from build123d import *

# Parameters (mm, degrees)
SKETCH1_R           = 50
BOSS_EXTRUDE1_DEPTH = 7
SKETCH2_R           = 2.5
BOSS_EXTRUDE2_DEPTH = 12.6
CIRPATTERN1_COUNT   = 12
SKETCH3_R           = 12
CUT_EXTRUDE1_DEPTH  = 8
SKETCH4_R           = 31.5
SKETCH4_R_2         = 16.5
CUT_EXTRUDE2_DEPTH  = 3
BOSS_EXTRUDE3_START = -4.2
SKETCH5_R           = 12
SKETCH5_R_2         = 8.5
BOSS_EXTRUDE3_DEPTH = 2.8


with BuildPart() as part:
    # Sketch1 → Boss-Extrude1 (new body)
    with BuildSketch(Plane.XY):
        Circle(SKETCH1_R)
    extrude(amount=-BOSS_EXTRUDE1_DEPTH)

    # Sketch2 → Boss-Extrude2 (add)
    with BuildSketch(Plane.XY):
        with BuildLine():
            Line((44.72775, 4.942507454), (48.490092946, 5.358254011))
            ThreePointArc((48.490092946, 5.358254011), (49.383550497, 5.092810123), (49.817513468, 4.267944684))
            ThreePointArc((49.817513468, 4.267944684), (50, 0), (49.817513468, -4.267944684))
            ThreePointArc((49.817513468, -4.267944684), (49.383550497, -5.092810123), (48.490092946, -5.358254011))
            Line((48.490092946, -5.358254011), (44.72775, -4.942507454))
            ThreePointArc((44.72775, -4.942507454), (40.05, 0), (44.72775, 4.942507454))
        make_face()
        with Locations((45, 0)):
            Circle(SKETCH2_R, mode=Mode.SUBTRACT)
    boss_extrude2 = extrude(amount=BOSS_EXTRUDE2_DEPTH)

    # CirPattern1: Boss-Extrude2 ×12 about axis
    cirpattern1_axis = Axis((0, 0, 0), (0, 0, 1))
    for i in range(1, CIRPATTERN1_COUNT):
        add(boss_extrude2.rotate(cirpattern1_axis, i * 360 / CIRPATTERN1_COUNT))

    # Sketch3 → Cut-Extrude1 (cut, through all)
    with BuildSketch(Plane.XY):
        Circle(SKETCH3_R)
    extrude(amount=-CUT_EXTRUDE1_DEPTH, mode=Mode.SUBTRACT)

    # Sketch4 → Cut-Extrude2 (cut)
    with BuildSketch(Plane.XY):
        Circle(SKETCH4_R)
        Circle(SKETCH4_R_2, mode=Mode.SUBTRACT)
    extrude(amount=-CUT_EXTRUDE2_DEPTH, mode=Mode.SUBTRACT)

    # Sketch5 → Boss-Extrude3 (add)
    with BuildSketch(Plane.XY.offset(BOSS_EXTRUDE3_START)):
        Circle(SKETCH5_R)
        Circle(SKETCH5_R_2, mode=Mode.SUBTRACT)
    extrude(amount=-BOSS_EXTRUDE3_DEPTH)


solid = part.part
Can you work these out from the model? Positions are in its coordinate system, mm. A direction names the side the tool comes from. Give positions to 0.01 mm unless a question says otherwise; leave off trailing zeros. Order: outer loops, then holes, each group sorted by start corner. A loop starts at its lowest first (then second) coordinate and runs counter-clockwise, first axis right, second up. Notation, with made-up numbers: (60, -1.5) - (73, -1.5) arc R12 cw to (73, 7.5) - close; hole circle Ø5 at (73.5, 4). An arc over 180 degrees is marked (long way). Write each question's results on one line, items separated by ' | '.
1) Please list where these lines run through material, in increasing order: line 1 along Y through (x, z) = (0, -2); line 2 along X through (y, z) = (22.5, 3.75). Write a range as [from, to].
Final values:
line 1: y = [-50, -31.5], [-16.5, -12], [12, 16.5], [31.5, 50] | line 2: x = [-44.65, -41.47], [-36.47, -34.02], [34.02, 36.47], [41.47, 44.65]
2) Suppose I cut it at B-B, the plane z = 6.5. Give the number of separate pieces and of enclosed holes in the cut face, then the cut area to 3 significant figures.
Final values:
separate pieces: 12 | enclosed holes: 12 | area: 835 mm^2
3) On a 3-axis mill with a long thin cutter (end or side, diameter ignored), from which of +Z, -Z, +X, -X, +Y, -Y can I reach the whole of each face in a straight line? I mean faces 4 (the face through (-37.81, 27.78, 6.21)), 5 (the face through (-23, 42, 12.6)), 6 (the face through (42.915, -18.833, 6.212)), 7 (the face through (1.15, -12.15, 0)). Say none if no direction works.
Final values:
face 4: +Z, +Y | face 5: +Z, +X, -X, +Y, -Y | face 6: +Z, +X | face 7: +Z
4) Suppose I cut it at C-C, the plane y = 22.5. Write out the boundary of the cut face in (x, z), then the cut area to 3 significant figures.
Final values:
outline: (-44.65, -7) - (44.65, -7) - (44.65, 12.6) - (41.47, 12.6) - (41.47, 0) - (36.47, 0) - (36.47, 12.6) - (34.02, 12.6) - (34.02, 0) - (22.05, 0) - (22.05, -3) - (-22.05, -3) - (-22.05, 0) - (-34.02, 0) - (-34.02, 12.6) - (-36.47, 12.6) - (-36.47, 0) - (-41.47, 0) - (-41.47, 12.6) - (-44.65, 12.6) - close | area: 635 mm^2
5) If we mould it in two halves opening along X, with no side actions, what happens to faces 1 (the face through (-25, -40, 12.6)), 2 (the face through (-0.96, -47.31, 6.21)), 3 (the face through (42.964, 18.855, 6.212))? For each: pulls with the +X half, pulls with the -X half, needs draft (parallel to the pull), parting line crosses it, or undercut.
Final values:
face 1: needs draft | face 2: undercut | face 3: pulls with the +X half
6) I'm going to push flat-ended pins straight in: pin 1 Ø5 at (y, z) = (-33.5, 8) entering from +X; pin 2 Ø5 at (y, z) = (23, -3) entering from +X; pin 3 Ø1.5 at (x, y) = (-0.5, 45) entering from +Z; pin 4 Ø6 at (y, z) = (13.5, 4.5) entering from -X. Where does each tip first touch, or does it pass through?
Final values:
pin 1: stops at x = 26.46 | pin 2: stops at x = 45.6 | pin 3: stops at z = 0 | pin 4: passes through
